```python
from build123d import *

# Parameters (mm, degrees)
F1_DEPTH  = 19.4
F2_R      = 3
F4_DEPTH  = 14.5
F5_R      = 3.25
F6_DEPTH  = 69.4177661804
F9_R      = 6.75
F10_DEPTH = 62.9177661804
F11_SIZE  = 2


with BuildPart() as f1:
    # F0 (on Top) → F1 (new body)
    with BuildSketch(Plane.XY):
        Polygon((-105, -39.9503339168), (-105, -44.9503339168), (105, -44.9503339168), (105, -39.9503339168), (40, 25.0496660832), align=None)
    extrude(amount=F1_DEPTH)

    # F2
    f2_edges = [f1.edges().sort_by_distance(p)[0] for p in [
        (40, 25.049666, 9.7),
        (105, -39.950334, 9.7),
        (-105, -39.950334, 9.7),
    ]]
    fillet(f2_edges, radius=F2_R)

    # F3 (on face) → F4 (cut)
    with BuildSketch(Plane.XZ.offset(44.9503339168)):
        with BuildLine():
            ThreePointArc((49.6338428976, 0), (54.0933027869, 3.9663846985), (55.75, 9.7))
            ThreePointArc((55.75, 9.7), (54.0933027869, 15.4336153015), (49.6338428976, 19.4))
            Line((49.6338428976, 19.4), (40.3661571024, 19.4))
            ThreePointArc((40.3661571024, 19.4), (34.25, 9.7), (40.3661571024, 0))
            Line((40.3661571024, 0), (49.6338428976, 0))
        make_face()
    extrude(amount=-F4_DEPTH, mode=Mode.SUBTRACT)

    # F5 (on face) → F6 (cut, through all)
    with BuildSketch(Plane.XZ.offset(44.9503339168)):
        with Locations((-35, 9.7000030801)):
            Circle(F5_R)
        with Locations((85, 9.7000030801)):
            Circle(F5_R)
    extrude(amount=-F6_DEPTH, mode=Mode.SUBTRACT)

    # F9 (on offset) → F10 (cut, through all)
    with BuildSketch(Plane.XZ.offset(38.4503339168)):
        with Locations((85, 9.7000030801)):
            Circle(F9_R)
        with Locations((-35, 9.7000030801)):
            Circle(F9_R)
    extrude(amount=-F10_DEPTH, mode=Mode.SUBTRACT)

    # F11
    f11_edges = [f1.edges().sort_by_distance(p)[0] for p in [
        (-105, -43.421739, 19.4),
        (-104.518085, -40.262424, 19.4),
        (-32.556871, -7.475828, 19.4),
        (39.883553, 24.416889, 19.4),
        (72.791617, -7.741951, 19.4),
        (105, -43.071654, 19.4),
        (72.791617, -7.741951, 0),
    ]]
    chamfer(f11_edges, length=F11_SIZE)


solid = f1.part
```
For this review, take the finished solid that the model builds, in its own axes (mm). A direction names the side the tool comes from. Coordinates: 2 decimals unless noted, no trailing zeros. Write each loop counter-clockwise with the first axis right and the second up, starting at its lowest first coordinate (ties: lowest second). Pieces come first, ordered by that corner, then holes.
(1) Wall thickness on probe 1 along Z at (x, y) = (85, -28); probe 2 along X at (y, z) = (-30.5, 5.75); probe 3 along Z at (x, y) = (-35, -43): over which ranges is each line inside the solid? List them lowest first.
(2) Add section A-A on x = 85. Give the boundary of the cut face in (y, z), then the cut area to 3 significant figures.
(3) Tool access review of faces 4 (the face through (78.257, -28.701, 9.997)), 5 (the face through (45, -30.45, 10)), 6 (the face through (105, -43, 10)): name each direction out of +Z, -Z, +X, -X, +Y, -Y from which nothing blocks a thin tool from reaching the whole face with its end or side.
(4) Add section C-C on x = -35. Give the boundary of the cut face in (y, z), then the cut area to 3 significant figures.
(5) Add section B-B on y = -34.5. Give the boundary of the cut face in (x, z), then the cut area to 3 significant figures.
(6) The part is to be moulded in two halves that separate along X. For faces 1 (the face through (-34, -38.45, 13)), 2 (the face through (72.53, -8.88, 1.01)), 3 (the face through (-31.153, -7.958, 18.414)), say which applies: +X half, -X half, draft (parallel to the pull), parting line (faces both ways), or undercut.
(7) Add section D-D on y = 3.5. Give the boundary of the cut face in (x, z), then the cut area to 3 significant figures.
(8) For pin 1 Ø8 at (y, z) = (-11, 2.5) entering from +X; pin 2 Ø8.5 at (x, z) = (-35, 9.7) entering from +Y; pin 3 Ø4 at (y, z) = (16.5, 9) entering from +X, all flat-tipped, find the tip position at first contact; note any pin that passes through.
Answer sheet:
1. probe 1: z = 0 to 2.95, 16.45 to 19.4
1. probe 2: x = -83.92 to -40.47, -29.53 to 35, 55 to 79.53, 90.47 to 95.55
1. probe 3: z = 0 to 6.45, 12.95 to 19.4
2. outline: (-44.95, 0) - (-22.78, 0) - (-19.95, 2) - (-19.95, 2.95) - (-38.45, 2.95) - (-38.45, 6.45) - (-44.95, 6.45) - close; (-44.95, 12.95) - (-38.45, 12.95) - (-38.45, 16.45) - (-19.95, 16.45) - (-19.95, 17.4) - (-22.78, 19.4) - (-44.95, 19.4) - close
2. area: 187 mm2
3. face 4: +Y
3. face 5: -Y
3. face 6: +Z, -Z, +X, +Y, -Y
4. outline: (-44.95, 0) - (-10.76, 0) - (-8.57, 2) - (-8.57, 2.95) - (-38.45, 2.95) - (-38.45, 6.45) - (-44.95, 6.45) - close; (-44.95, 12.95) - (-38.45, 12.95) - (-38.45, 16.45) - (-8.57, 16.45) - (-8.57, 17.4) - (-10.76, 19.4) - (-44.95, 19.4) - close
4. area: 256 mm2
5. outline: (-92.84, 2) - (-87.95, 0) - (40.37, 0) arc R10.75 cw to (40.37, 19.4) - (-87.95, 19.4) - (-92.84, 17.4) - close; (49.63, 0) - (96.72, 0) - (99.55, 2) - (99.55, 17.4) - (96.72, 19.4) - (49.63, 19.4) arc R10.75 cw to start; hole circle Ø13.5 at (-35, 9.7); hole circle Ø13.5 at (85, 9.7)
5. area: 3,080 mm2
6. face 1: undercut
6. face 2: +X half
6. face 3: -X half
7. outline: (-8.07, 2) - (-3.18, 0) - (58.72, 0) - (61.55, 2) - (61.55, 17.4) - (58.72, 19.4) - (-3.18, 19.4) - (-8.07, 17.4) - close
7. area: 1,340 mm2
8. pin 1: stops at x = 80.05
8. pin 2: stops at y = -38.45
8. pin 3: stops at x = 50.55
